from build123d import *

# Parameters (mm, degrees)
REVOLVE001_PLACEMENT_ANGLE  = 330
REVOLVE002_PLACEMENT_ANGLE  = 330
REVOLVE003_PLACEMENT_ANGLE  = 330
REVOLVE_PLACEMENT_ANGLE     = 330
EXTRUDE008_DEPTH            = 2
EXTRUDE007_DEPTH            = 2
CYLINDER011_R               = 3.8
CYLINDER011_DEPTH           = 3
CYLINDER011_PLACEMENT_ANGLE = 60
BOX020_W                    = 73.2
BOX020_H                    = 27.2
BOX020_DEPTH                = 3
BOX020_PLACEMENT_ANGLE      = 60
EXTRUDE006_DEPTH            = 140
FILLET013_R                 = 1
FILLET014_R                 = 1


with BuildPart() as revolve001:
    # Sketch040 → Revolve001 (revolve)
    with BuildSketch(Plane.YZ):
        with BuildLine():
            Line((0, 0), (0, 2.3))
            Line((0, 2.3), (8.5, 2.3))
            Line((8.5, 2.3), (8.5, 1.35))
            Line((8.5, 1.35), (5.1, 1.35))
            ThreePointArc((5.1, 1.35), (3.75, 1.75), (2.4, 1.35))
            Line((1.4, 1.35), (2.4, 1.35))
            Line((1.4, 0), (1.4, 1.35))
            Line((0, 0), (1.4, 0))
        make_face()
    revolve(axis=Axis((0, 0, 0), (0, 1, 0)))


with BuildPart() as revolve001_1:
    # Revolve001 placement: moved
    add(revolve001.part.moved(Location((-21.009, -76.9733, -41.739))).rotate(Axis((-21.009, -76.9733, -41.739), (1, 0, 0)), REVOLVE001_PLACEMENT_ANGLE))


with BuildPart() as revolve002:
    # Sketch040 → Revolve002 (revolve)
    with BuildSketch(Plane.YZ):
        with BuildLine():
            Line((0, 0), (0, 2.3))
            Line((0, 2.3), (8.5, 2.3))
            Line((8.5, 2.3), (8.5, 1.35))
            Line((8.5, 1.35), (5.1, 1.35))
            ThreePointArc((5.1, 1.35), (3.75, 1.75), (2.4, 1.35))
            Line((1.4, 1.35), (2.4, 1.35))
            Line((1.4, 0), (1.4, 1.35))
            Line((0, 0), (1.4, 0))
        make_face()
    revolve(axis=Axis((0, 0, 0), (0, 1, 0)))


with BuildPart() as revolve002_1:
    # Revolve002 placement: moved
    add(revolve002.part.moved(Location((-21.009, -92.473316, -68.585836))).rotate(Axis((-21.009, -92.473316, -68.585836), (1, 0, 0)), REVOLVE002_PLACEMENT_ANGLE))


with BuildPart() as revolve003:
    # Sketch040 → Revolve003 (revolve)
    with BuildSketch(Plane.YZ):
        with BuildLine():
            Line((0, 0), (0, 2.3))
            Line((0, 2.3), (8.5, 2.3))
            Line((8.5, 2.3), (8.5, 1.35))
            Line((8.5, 1.35), (5.1, 1.35))
            ThreePointArc((5.1, 1.35), (3.75, 1.75), (2.4, 1.35))
            Line((1.4, 1.35), (2.4, 1.35))
            Line((1.4, 0), (1.4, 1.35))
            Line((0, 0), (1.4, 0))
        make_face()
    revolve(axis=Axis((0, 0, 0), (0, 1, 0)))


with BuildPart() as revolve003_1:
    # Revolve003 placement: moved
    add(revolve003.part.moved(Location((53.991, -92.4733, -68.5858))).rotate(Axis((53.991, -92.4733, -68.5858), (1, 0, 0)), REVOLVE003_PLACEMENT_ANGLE))


with BuildPart() as revolve_body:
    # Sketch040 → Revolve (revolve)
    with BuildSketch(Plane.YZ):
        with BuildLine():
            Line((0, 0), (0, 2.3))
            Line((0, 2.3), (8.5, 2.3))
            Line((8.5, 2.3), (8.5, 1.35))
            Line((8.5, 1.35), (5.1, 1.35))
            ThreePointArc((5.1, 1.35), (3.75, 1.75), (2.4, 1.35))
            Line((1.4, 1.35), (2.4, 1.35))
            Line((1.4, 0), (1.4, 1.35))
            Line((0, 0), (1.4, 0))
        make_face()
    revolve(axis=Axis((0, 0, 0), (0, 1, 0)))


with BuildPart() as revolve_body_1:
    # Revolve placement: moved
    add(revolve_body.part.moved(Location((53.991, -76.973316, -41.739049))).rotate(Axis((53.991, -76.973316, -41.739049), (1, 0, 0)), REVOLVE_PLACEMENT_ANGLE))


with BuildPart() as extrude008:
    # Sketch032 → Extrude008 (new body)
    with BuildSketch(Plane.YZ):
        with BuildLine():
            Line((0, 0), (-43.366025, 0))
            ThreePointArc((-44.665064, 2.25), (-44.665064, 0.75), (-43.366025, 0))
            Line((-44.665064, 2.25), (-22.165064, 41.221143))
            ThreePointArc((-20, 42.471143), (-21.25, 42.136207), (-22.165064, 41.221143))
            Line((-20, 42.471143), (0, 42.471143))
            Line((0, 42.471143), (0, 40))
            Line((0, 40), (6.4, 40))
            Line((6.4, 40), (6.4, 34))
            ThreePointArc((3.4, 34), (4.9, 32.5), (6.4, 34))
            Line((3.4, 36), (3.4, 34))
            Line((0, 36), (3.4, 36))
            Line((0, 36), (0, 12))
            Line((6.4, 12), (0, 12))
            Line((6.4, 6), (6.4, 12))
            ThreePointArc((3.4, 6), (4.9, 4.5), (6.4, 6))
            Line((3.4, 8), (3.4, 6))
            Line((0, 8), (3.4, 8))
            Line((0, 0), (0, 8))
        make_face()
    extrude(amount=EXTRUDE008_DEPTH)


with BuildPart() as extrude008_1:
    # Extrude008 placement: moved
    add(extrude008.part.moved(Location((-70.558895, -50.039221, -79.500001))))


with BuildPart() as extrude007:
    # Sketch032 → Extrude007 (new body)
    with BuildSketch(Plane.YZ):
        with BuildLine():
            Line((0, 0), (-43.366025, 0))
            ThreePointArc((-44.665064, 2.25), (-44.665064, 0.75), (-43.366025, 0))
            Line((-44.665064, 2.25), (-22.165064, 41.221143))
            ThreePointArc((-20, 42.471143), (-21.25, 42.136207), (-22.165064, 41.221143))
            Line((-20, 42.471143), (0, 42.471143))
            Line((0, 42.471143), (0, 40))
            Line((0, 40), (6.4, 40))
            Line((6.4, 40), (6.4, 34))
            ThreePointArc((3.4, 34), (4.9, 32.5), (6.4, 34))
            Line((3.4, 36), (3.4, 34))
            Line((0, 36), (3.4, 36))
            Line((0, 36), (0, 12))
            Line((6.4, 12), (0, 12))
            Line((6.4, 6), (6.4, 12))
            ThreePointArc((3.4, 6), (4.9, 4.5), (6.4, 6))
            Line((3.4, 8), (3.4, 6))
            Line((0, 8), (3.4, 8))
            Line((0, 0), (0, 8))
        make_face()
    extrude(amount=EXTRUDE007_DEPTH)


with BuildPart() as extrude007_1:
    # Extrude007 placement: moved
    add(extrude007.part.moved(Location((67.441105, -50.039221, -79.500001))))


with BuildPart() as cylinder011:
    # Cylinder011 → Cylinder011 (new body)
    with BuildSketch(Plane.XY):
        Circle(CYLINDER011_R)
    extrude(amount=CYLINDER011_DEPTH)


with BuildPart() as cylinder011_1:
    # Cylinder011 placement: moved
    add(cylinder011.part.moved(Location((25, -10.2958, 29.038294))).rotate(Axis((25, -10.2958, 29.038294), (1, 0, 0)), CYLINDER011_PLACEMENT_ANGLE))


with BuildPart() as cube004:
    # Box020 → Box020 (new body)
    with BuildSketch(Plane.XY):
        with Locations((36.6, 13.6)):
            Rectangle(BOX020_W, BOX020_H)
    extrude(amount=BOX020_DEPTH)


with BuildPart() as cube004_1:
    # Box020 placement: moved
    add(cube004.part.moved(Location((51, -19.2958, 13.449837))).rotate(Axis((51, -19.2958, 13.449837), (1, 0, 0)), BOX020_PLACEMENT_ANGLE))


with BuildPart() as fusion010:
    # Sketch031 → Extrude006 (new body)
    with BuildSketch(Plane.YZ):
        with BuildLine():
            Line((20, 47.471143), (0, 47.471143))
            ThreePointArc((0, 47.471143), (-2.5, 46.80127), (-4.330127, 44.971143))
            Line((-4.330127, 44.971143), (-26.830127, 6))
            ThreePointArc((-26.830127, 6), (-26.830127, 2), (-23.366025, 0))
            Line((-23.366025, 0), (20, 0))
            Line((20, 0), (20, 2.5))
            Line((20, 2.5), (-23.366025, 2.5))
            ThreePointArc((-24.665064, 4.75), (-24.665064, 3.25), (-23.366025, 2.5))
            Line((-24.665064, 4.75), (-2.165064, 43.721143))
            ThreePointArc((0, 44.971143), (-1.25, 44.636207), (-2.165064, 43.721143))
            Line((0, 44.971143), (20, 44.971143))
            Line((20, 44.971143), (20, 47.471143))
        make_face()
    extrude(amount=EXTRUDE006_DEPTH)

    # Cut003: cut Cube004
    add(cube004_1.part, mode=Mode.SUBTRACT)

    # Cut004: cut Cylinder011
    add(cylinder011_1.part, mode=Mode.SUBTRACT)


with BuildPart() as fusion010_1:
    # Cut004 placement: moved
    add(fusion010.part.moved(Location((-70.558895, -70.039221, -82.000001))))

    # Fillet013
    fillet013_edges = [fusion010_1.edges().sort_by_distance(p)[0] for p in [
        (69.441105, -60.039221, -34.528858),
        (69.441105, -72.539221, -35.198731),
        (69.441105, -85.619348, -56.514429),
        (69.441105, -96.869348, -80.000001),
        (69.441105, -71.722234, -82.000001),
    ]]
    fillet(fillet013_edges, radius=FILLET013_R)

    # Fillet014
    fillet014_edges = [fusion010_1.edges().sort_by_distance(p)[0] for p in [
        (-70.558895, -60.039221, -34.528858),
        (-70.558895, -72.539221, -35.198731),
        (-70.558895, -85.619348, -56.514429),
        (-70.558895, -96.869348, -80.000001),
        (-70.558895, -71.722234, -82.000001),
    ]]
    fillet(fillet014_edges, radius=FILLET014_R)

    # Fusion005: union Extrude007
    add(extrude007_1.part)

    # Fusion006: union Extrude008
    add(extrude008_1.part)

    # Fusion007: union Revolve body
    add(revolve_body_1.part)

    # Fusion008: union Revolve003
    add(revolve003_1.part)

    # Fusion009: union Revolve002
    add(revolve002_1.part)

    # Fusion010: union Revolve001
    add(revolve001_1.part)


solid = fusion010_1.part
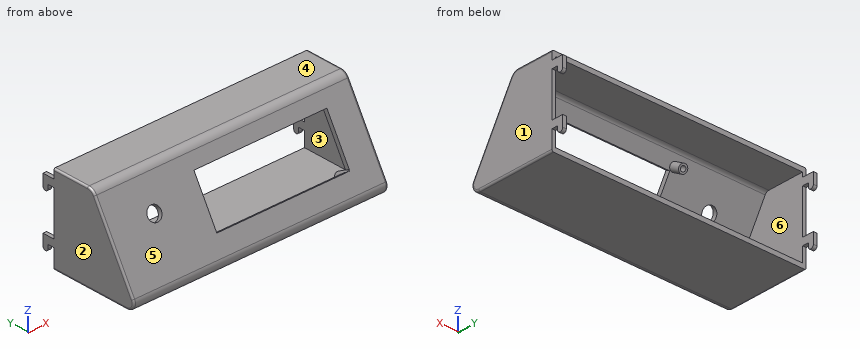
Here's how the part is built. I have some questions about the finished solid (model axes, mm). Face numbers are marked on the shaded views. A direction names the side the tool comes from. Coordinates: 2 decimals unless noted, no trailing zeros. Order: outer loops, then holes, each group sorted by start corner. A loop starts at its lowest first (then second) coordinate and runs counter-clockwise, first axis right, second up. Notation, with made-up numbers: M -7,-32 L 9,-32 A23 ccw 9,-20 Z; hole C 79,-8 d1. An arc over 180 degrees is marked long. Answer as CSV lines item,"result". Start each with the question number.
1. I want a section at C-C, the plane x = -38.5. Write out the boundary of the cut face in (y, z).
2. I want a section at A-A, the plane x = -10.5. Write out the boundary of the cut face in (y, z), and give its area (3 significant figures).
3. I need wall thicknesses on line 1 (Z direction, x = 30.5, y = -67.5); line 2 (X direction, y = -70, z = -51.5); line 3 (Z direction, x = 20, y = -71.5). Which ranges of each line are inside material? Lowest first, please. Write a range as [from, to].
4. For pin 1 (1.6 mm diameter, centred on x = -69, z = -44.5, fed in from -Y); pin 2 (0.6 mm diameter, centred on x = 68, z = -51, fed in from +Y); pin 3 (2 mm diameter, centred on x = -69.5, y = -49, fed in from -Z), each with a flat end and sliding along its axis, tell me the tip position at first contact or that it passes through.
5. I want a section at B-B, the plane y = -67. Write out the boundary of the cut face in (x, z), and give its area (3 significant figures).
6. We'd pull the mould along X, two halves only. Please class the marked faces 1, 2, 3 and 4: released by +X, released by -X, zero draft, split by the parting line, or undercut.
7. On a 3-axis mill with a long thin cutter (end or side, diameter ignored), from which of +Z, -Z, +X, -X, +Y, -Y can I reach the whole of each face in a straight line? I mean the marked faces 5 and 6. Say none if no direction works.
Recorded:
1,outline,"M -96.87,-76 A4 ccw -93.41,-82 L -50.04,-82 L -50.04,-79.5 L -93.41,-79.5 A1.5 cw -94.7,-77.25 L -72.2,-38.28 A2.5 cw -70.04,-37.03 L -50.04,-37.03 L -50.04,-34.53 L -70.04,-34.53 A5 ccw -74.37,-37.03 Z"
2,outline,"M -96.87,-76 A4 ccw -93.41,-82 L -50.04,-82 L -50.04,-79.5 L -93.41,-79.5 A1.5 cw -94.7,-77.25 L -89.59,-68.4 L -91.76,-67.15 Z; M -78.16,-43.59 L -75.99,-44.84 L -72.2,-38.28 A2.5 cw -70.04,-37.03 L -50.04,-37.03 L -50.04,-34.53 L -70.04,-34.53 A5 ccw -74.37,-37.03 Z"
2,area,"227 mm2"
3,line 1,"z = [-82, -79.5], [-37.03, -34.53]"
3,line 2,"x = [-70.56, -68.56], [67.44, 69.44]"
3,line 3,"z = [-82, -79.5], [-37.5, -34.75]"
4,pin 1,"stops at y = -79.14"
4,pin 2,"stops at y = -50.04"
4,pin 3,"stops at z = -71.5"
5,outline,"M -70.56,-81 A1 ccw -69.56,-82 L 68.44,-82 A1 ccw 69.44,-81 L 69.44,-35.53 A1 ccw 68.44,-34.53 L -69.56,-34.53 A1 ccw -70.56,-35.53 Z; hole M -68.56,-79.5 L 67.44,-79.5 L 67.44,-37.03 L -68.56,-37.03 Z"
5,area,"869 mm2"
6,face 1,"released by +X"
6,face 2,"released by -X"
6,face 3,"undercut"
6,face 4,"zero draft"
7,face 5,"+Z, +X, -X, -Y"
7,face 6,"+Y"
